Here's how the part is built. I have some questions about the finished solid (model axes, mm). A direction names the side the tool comes from. Coordinates: 2 decimals unless noted, no trailing zeros. Write each loop counter-clockwise with the first axis right and the second up, starting at its lowest first coordinate (ties: lowest second). Pieces come first, ordered by that corner, then holes. Notation, with made-up numbers: (73, 29.5) -> (79, 29.5) arc R12 cw to (79, 35.5) -> close; hole circle Ø1 at (31.25, 81.5). An arc over 180 degrees is marked (long way). Put each result on its own line as item: value.
```python
from build123d import *

# Parameters (mm, degrees)
F1_DEPTH = 4
F2_W     = 2
F2_H     = 7.5
F3_DEPTH = 1.7
F5_DEPTH = 10
F6_R     = 1
F7_DEPTH = 25


with BuildPart() as f1:
    # F0 (on Top) → F1 (new body)
    with BuildSketch(Plane.XY):
        with BuildLine():
            Line((6, 0), (55, 0))
            Line((55, 0), (55, -9))
            ThreePointArc((55, -9), (58, -12), (61, -9))
            Line((61, -9), (61, 19))
            ThreePointArc((61, 19), (58, 22), (55, 19))
            Line((55, 19), (55, 10))
            Line((55, 10), (50, 10))
            Line((50, 10), (50, 2.5))
            Line((50, 2.5), (38.5, 2.5))
            Line((38.5, 2.5), (38.5, 10))
            Line((38.5, 10), (20.5, 10))
            Line((20.5, 10), (20.5, 2.5))
            Line((20.5, 2.5), (9, 2.5))
            Line((9, 2.5), (9, 10))
            Line((9, 10), (6, 10))
            Line((6, 10), (6, 19))
            ThreePointArc((6, 19), (3, 22), (0, 19))
            Line((0, 19), (0, -9))
            ThreePointArc((0, -9), (3, -12), (6, -9))
            Line((6, -9), (6, 0))
        make_face()
    extrude(amount=F1_DEPTH)

    # F2 (on Top) → F3 (join)
    with BuildSketch(Plane.XY):
        with Locations((12, 6.25)):
            Rectangle(F2_W, F2_H)
        with Locations((17.5, 6.25)):
            Rectangle(F2_W, F2_H)
        with Locations((41.5, 6.25)):
            Rectangle(F2_W, F2_H)
        with Locations((47, 6.25)):
            Rectangle(F2_W, F2_H)
    extrude(amount=F3_DEPTH)

    # F4 (on face) → F5 (join)
    with BuildSketch(Plane.XY.offset(4)):
        with BuildLine():
            ThreePointArc((0, 19), (3, 16), (6, 19))
            ThreePointArc((6, 19), (3, 22), (0, 19))
        make_face()
        with BuildLine():
            ThreePointArc((6, -9), (3, -6), (0, -9))
            ThreePointArc((0, -9), (3, -12), (6, -9))
        make_face()
        with BuildLine():
            ThreePointArc((61, -9), (58, -6), (55, -9))
            ThreePointArc((55, -9), (58, -12), (61, -9))
        make_face()
        with BuildLine():
            ThreePointArc((55, 19), (58, 16), (61, 19))
            ThreePointArc((61, 19), (58, 22), (55, 19))
        make_face()
    extrude(amount=F5_DEPTH)

    # F6 (on face) → F7 (cut)
    with BuildSketch(Plane(origin=(0, 0, 0), x_dir=(1, 0, 0), z_dir=(0, 0, -1))):
        with Locations((3, 9)):
            Circle(F6_R)
        with Locations((58, 9)):
            Circle(F6_R)
        with Locations((58, -19)):
            Circle(F6_R)
        with Locations((3, -19)):
            Circle(F6_R)
    extrude(amount=-F7_DEPTH, mode=Mode.SUBTRACT)


solid = f1.part
```
Item 1: Imagine slicing it at D-D on x = 22. Write out the boundary of the cut face in (y, z).
Output:
outline: (0, 0) -> (10, 0) -> (10, 4) -> (0, 4) -> close
Item 2: For P1, Ø3, axis at y = 15, z = 3, coming from the -X side; P2, Ø1, axis at x = 42, y = 7, coming from the +Z side; P3, Ø5, axis at x = 35.5, z = 5, coming from the -Y side; P4, Ø1.9, axis at x = 12.5, z = 1, coming from the +Y side, each with a flat end and sliding along its axis, tell me the tip position at first contact or that it passes through.
Output:
P1: stops at x = 0
P2: stops at z = 1.7
P3: stops at y = 0
P4: stops at y = 10
Item 3: Please list where these lines run through material, in increasing order: line 1 along X through (y, z) = (19, 3.75); line 2 along Y through (x, z) = (3, 5.25); line 3 along X through (y, z) = (-2.5, 3). Write a range as from..to.
Output:
line 1: x = 0..2, 4..6, 55..57, 59..61
line 2: y = -12..-10, -8..-6, 16..18, 20..22
line 3: x = 0..6, 55..61
Item 4: Imagine slicing it at A-A on z = 11.5. Write out the boundary of the cut face in (x, y).
Output:
outline: circle Ø6 at (3, -9); circle Ø6 at (3, 19); circle Ø6 at (58, -9); circle Ø6 at (58, 19); hole circle Ø2 at (3, -9); hole circle Ø2 at (3, 19); hole circle Ø2 at (58, -9); hole circle Ø2 at (58, 19)
Item 5: Imagine slicing it at B-B on y = 6.5. Write out the boundary of the cut face in (x, z).
Output:
outline: (0, 0) -> (9, 0) -> (9, 4) -> (0, 4) -> close; (11, 0) -> (13, 0) -> (13, 1.7) -> (11, 1.7) -> close; (16.5, 0) -> (18.5, 0) -> (18.5, 1.7) -> (16.5, 1.7) -> close; (20.5, 0) -> (38.5, 0) -> (38.5, 4) -> (20.5, 4) -> close; (40.5, 0) -> (42.5, 0) -> (42.5, 1.7) -> (40.5, 1.7) -> close; (46, 0) -> (48, 0) -> (48, 1.7) -> (46, 1.7) -> close; (50, 0) -> (61, 0) -> (61, 4) -> (50, 4) -> close
Item 6: Imagine slicing it at C-C on x = 58. Write out the boundary of the cut face in (y, z).
Output:
outline: (-12, 0) -> (-10, 0) -> (-10, 14) -> (-12, 14) -> close; (-8, 0) -> (18, 0) -> (18, 14) -> (16, 14) -> (16, 4) -> (-6, 4) -> (-6, 14) -> (-8, 14) -> close; (20, 0) -> (22, 0) -> (22, 14) -> (20, 14) -> close
Item 7: If we mould it in two halves opening along X, with no side actions, what happens to faces 5 (the flat face through (17, 6, 1.7)), 6 (the flat face through (2, -8, 14))? For each: released by +X, released by -X, zero draft, split by the parting line, or undercut.
Output:
face 5: undercut
face 6: zero draft
Item 8: Which directions (+Z, -Z, +X, -X, +Y, -Y) give clear straight access to the entire face, cutting with the end or side of a thin tool? Please do faces 1 (the flat face through (12, 6, 1.7)), 2 (the flat face through (55, -4, 2)), 3 (the cylindrical face through (3, -12, 8)), 4 (the flat face through (46, 6, 1)).
Output:
face 1: +Z, +Y
face 2: +Z, -Z, -Y
face 3: +Z
face 4: +Z, -Z, +Y
